Read the model definition and answer for the solid it produces. Units are mm, in the model's axes. Coordinates: 2 decimals unless noted, no trailing zeros. Loops run counter-clockwise (first coordinate to the right, second up) from the corner with the lowest first, then second, coordinate; pieces in that order, holes last. Notation, with made-up numbers: (16.5, 54) -> (51.5, 54) arc R20 ccw to (51.5, 60) -> close; hole circle Ø11 at (39, -8.75). An arc over 180 degrees is marked (long way). Answer in a Markdown table with one row per item.
```python
from build123d import *

# Parameters (mm, degrees)
F0_R     = 130
F1_DEPTH = 85
F3_D     = 20
F3_DEPTH = 85
F4_R     = 42


with BuildPart() as f1:
    # F0 (on Right) → F1 (new body)
    with BuildSketch(Plane.YZ):
        Circle(F0_R)
    extrude(amount=F1_DEPTH)

    # F3
    with Locations(Plane.YZ.offset(85)):
        with Locations((0, 0)):
            Hole(F3_D / 2, depth=F3_DEPTH)

    # F4
    f4_edges = [f1.edges().sort_by_distance(p)[0] for p in [
        (0, -130, 0),
        (85, -130, 0),
    ]]
    fillet(f4_edges, radius=F4_R)


solid = f1.part
```
1. A cutting plane is placed at C-C on x = 26. Give the vertices of the cut face in (y, z).
A:
| item | result |
|---|---|
| outline | circle Ø253.67 at (0, 0); hole circle Ø20 at (0, 0) |
2. Given pin 1 Ø8 at (x, y) = (46.5, -86.5) entering from -Z; pin 2 Ø5 at (x, z) = (76, -14) entering from -Y; pin 3 Ø8 at (y, z) = (-70.5, -66.5) entering from +X, each flat-ended and moving along its own axis, determine where each tip first touches the part or whether it passes through.
A:
| item | result |
|---|---|
| pin 1 | stops at z = -100.3 |
| pin 2 | stops at y = -116.05 |
| pin 3 | stops at x = 84.71 |
3. Find the intervals of material crossed by probe 1 along Z at (x, y) = (41, 0); probe 2 along X at (y, z) = (30, 84); probe 3 along Y at (x, z) = (41.5, -8.5), in increasing order.
A:
| item | result |
|---|---|
| probe 1 | z = -129.99 to -10, 10 to 129.99 |
| probe 2 | x = 0.02 to 84.98 |
| probe 3 | y = -129.72 to -5.27, 5.27 to 129.72 |
4. A cutting plane is placed at D-D on x = 67.5. Give the vertices of the cut face in (y, z).
A:
| item | result |
|---|---|
| outline | circle Ø244.23 at (0, 0); hole circle Ø20 at (0, 0) |
5. A cutting plane is placed at A-A on z = 0. Give the vertices of the cut face in (x, y).
A:
| item | result |
|---|---|
| outline | (0, -88) arc R42 ccw to (42, -130) -> (43, -130) arc R42 ccw to (85, -88) -> (85, -10) -> (0, -10) -> close; (0, 10) -> (85, 10) -> (85, 88) arc R42 ccw to (43, 130) -> (42, 130) arc R42 ccw to (0, 88) -> close |
6. The mould has two halves that part along Y. Classify faces 1 (the cylindrical face through (42.493, 123.997, 39.048)), 2 (the flat face through (85, -1, -18)), 3 (the cylindrical face through (41.9, 2.17, -9.76)): pulls with the +Y half, pulls with the -Y half, needs draft (parallel to the pull), parting line crosses it, or undercut.
A:
| item | result |
|---|---|
| face 1 | parting line crosses it |
| face 2 | needs draft |
| face 3 | undercut |
